Can you work these out from the drawing? Everything is in mm from the part's minimum corner. Coordinates: 2 decimals unless noted, no trailing zeros. Write each loop counter-clockwise with the first axis right and the second up, starting at its lowest first coordinate (ties: lowest second). Pieces come first, ordered by that corner, then holes.
(1) Imagine slicing it at D-D, the plane x = 6.5. List the corners of the cut face in (y, z) for me.
(2) Please list where these lines run through material, in increasing order: probe 1 along Z at (x, y) = (6.5, 45.3); probe 2 along X at (y, z) = (45, 35); probe 3 along Y at (x, z) = (34, 4.25).
(3) Thinking about a two-plate mould opening in Z: for the marked faces 1, 2 and 3, which applies, released by +Z, released by -Z, zero draft, split by the parting line, or undercut?
(4) Imagine slicing it at C-C, the plane z = 35. List the corners of the cut face in (x, y) for me.
(5) Imagine slicing it at A-A, the plane y = 26. List the corners of the cut face in (x, z) for me.
(6) For pin 1 Ø9.5 at (x, z) = (61.5, 35) entering from -Y; pin 2 Ø12 at (x, y) = (8, 9.5) entering from +Z, each with a flat end and sliding along its axis, tell me the tip position at first contact or that it passes through.
(7) Imagine slicing it at B-B, the plane x = 34. List the corners of the cut face in (y, z) for me, plus the area to 3 significant figures.
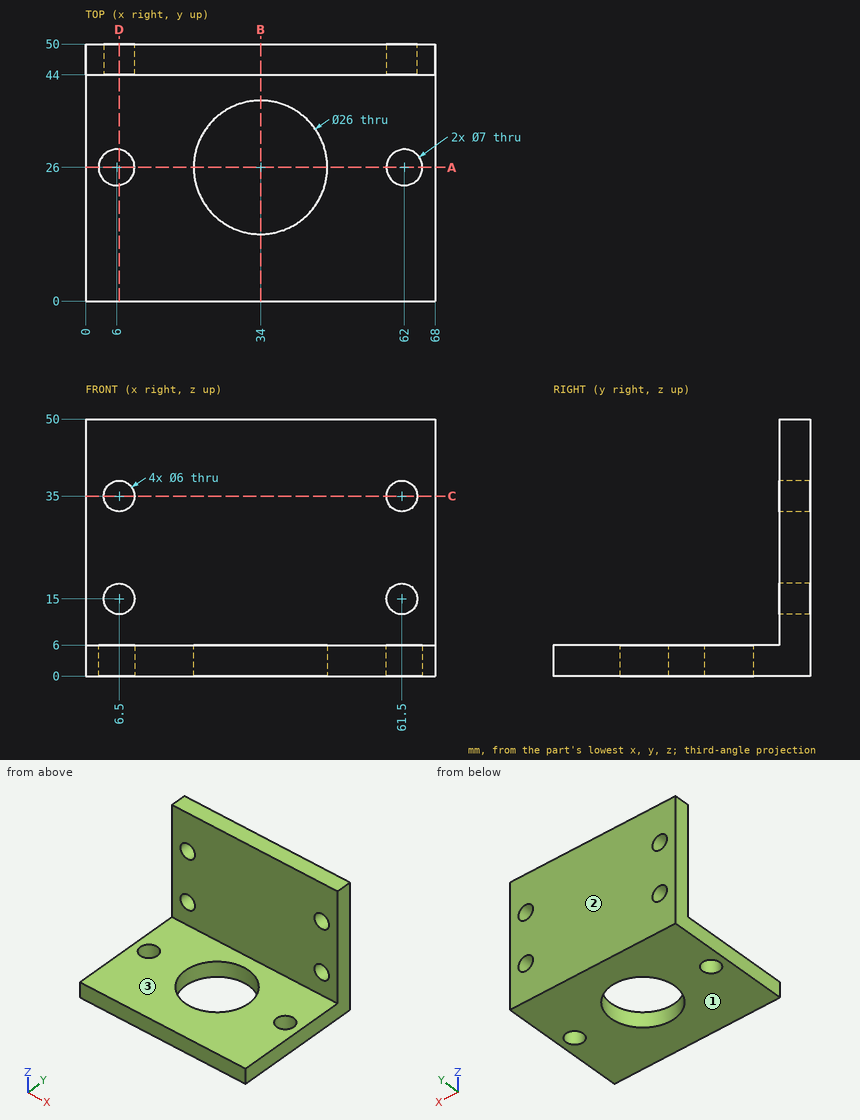
Recorded:
1. outline: (0, 0) - (22.54, 0) - (22.54, 6) - (0, 6) - close; (29.46, 0) - (50, 0) - (50, 12) - (44, 12) - (44, 6) - (29.46, 6) - close; (44, 18) - (50, 18) - (50, 32) - (44, 32) - close; (44, 38) - (50, 38) - (50, 50) - (44, 50) - close
2. probe 1: z = 0 to 12, 18 to 32, 38 to 50
2. probe 2: x = 0 to 3.5, 9.5 to 58.5, 64.5 to 68
2. probe 3: y = 0 to 13, 39 to 50
3. face 1: released by -Z
3. face 2: zero draft
3. face 3: released by +Z
4. outline: (0, 44) - (3.5, 44) - (3.5, 50) - (0, 50) - close; (9.5, 44) - (58.5, 44) - (58.5, 50) - (9.5, 50) - close; (64.5, 44) - (68, 44) - (68, 50) - (64.5, 50) - close
5. outline: (0, 0) - (2.5, 0) - (2.5, 6) - (0, 6) - close; (9.5, 0) - (21, 0) - (21, 6) - (9.5, 6) - close; (47, 0) - (58.5, 0) - (58.5, 6) - (47, 6) - close; (65.5, 0) - (68, 0) - (68, 6) - (65.5, 6) - close
6. pin 1: stops at y = 44
6. pin 2: stops at z = 6
7. outline: (0, 0) - (13, 0) - (13, 6) - (0, 6) - close; (39, 0) - (50, 0) - (50, 50) - (44, 50) - (44, 6) - (39, 6) - close
7. area: 408 mm2
